Check sheet for the modelled part. Datum: model origin and axes. Units: mm. A direction names the side the tool comes from. Round coordinates to 2 decimals unless told otherwise and drop trailing zeros. Loops run counter-clockwise (first coordinate to the right, second up) from the corner with the lowest first, then second, coordinate; pieces in that order, holes last. Notation, with made-up numbers: (-6.5, 74) -> (31.5, 74) arc R22 cw to (31.5, 87) -> close; hole circle Ø5 at (15.5, 65). An arc over 180 degrees is marked (long way). One line per question, with ' | ' between items.
```python
from build123d import *

# Parameters (mm, degrees)
F1_DEPTH  = 104.648
F2_W      = 6.35
F2_H      = 4.826
F3_DEPTH  = 28.575
F5_DEPTH  = 68.58
F7_DEPTH  = 12.7
F11_DEPTH = 39.116
F12_W     = 31.242
F12_H     = 31.75
F13_DEPTH = 67.31


with BuildPart() as f1:
    # F0 (on Right) → F1 (new body)
    with BuildSketch(Plane.YZ):
        Polygon((-14.224, 15.875), (-14.224, 0), (-14.224, -15.875), (-7.874, -15.875), (-7.874, -44.45), (7.874, -44.45), (7.874, -15.875), (14.224, -15.875), (14.224, 0), (14.224, 15.875), (7.874, 15.875), (7.874, 44.45), (-7.874, 44.45), (-7.874, 15.875), align=None)
    extrude(amount=-F1_DEPTH)

    # F2 (on face) → F3 (cut, through all)
    with BuildSketch(Plane.XY.offset(44.45)):
        with Locations((-101.473, -5.461)):
            Rectangle(F2_W, F2_H)
    extrude(amount=-F3_DEPTH, mode=Mode.SUBTRACT)

    # F4 (on Front) → F5 (cut, symmetric)
    with BuildSketch(Plane.XZ):
        with BuildLine():
            Line((-50.546, -24.638), (-74.422, -24.638))
            ThreePointArc((-74.422, -24.638), (-80.01, -30.226), (-74.422, -35.814))
            Line((-74.422, -35.814), (-50.546, -35.814))
            ThreePointArc((-50.546, -35.814), (-44.958, -30.226), (-50.546, -24.638))
        make_face()
        with BuildLine():
            ThreePointArc((-74.422, 35.814), (-80.01, 30.226), (-74.422, 24.638))
            Line((-74.422, 24.638), (-50.546, 24.638))
            ThreePointArc((-50.546, 24.638), (-44.958, 30.226), (-50.546, 35.814))
            Line((-50.546, 35.814), (-74.422, 35.814))
        make_face()
    extrude(amount=F5_DEPTH, both=True, mode=Mode.SUBTRACT)


with BuildPart() as f7:
    # F6 (on Front) → F7 (new body, symmetric)
    with BuildSketch(Plane.XZ):
        Polygon((0, 44.45), (-35.052, 44.45), (-35.052, 26.924), (-17.526, 26.924), align=None)
        Polygon((0, -44.45), (-17.526, -26.924), (-35.052, -26.924), (-35.052, -44.45), align=None)
    extrude(amount=F7_DEPTH, both=True)

    # F8: union F1
    add(f1.part)

    # F10 (on Front) → F11 (cut, symmetric)
    with BuildSketch(Plane.XZ):
        Polygon((0, 44.45), (-17.526, 26.924), (-28.575, 15.875), (0, 15.875), align=None)
        Polygon((-28.575, -15.875), (-17.526, -26.924), (0, -44.45), (0, -15.875), align=None)
    extrude(amount=F11_DEPTH, both=True, mode=Mode.SUBTRACT)

    # F12 (on Front) → F13 (cut, symmetric)
    with BuildSketch(Plane.XZ):
        with Locations((-15.621, 0)):
            Rectangle(F12_W, F12_H)
    extrude(amount=F13_DEPTH, both=True, mode=Mode.SUBTRACT)


solid = f7.part
```
(1) Sectioned sample at D-D, the plane x = -12.5. Record the cut outline in (y, z).
Answer:
outline: (-12.7, -44.45) -> (12.7, -44.45) -> (12.7, -31.95) -> (-12.7, -31.95) -> close; (-12.7, 31.95) -> (12.7, 31.95) -> (12.7, 44.45) -> (-12.7, 44.45) -> close
(2) Mould release check, pull along X, two halves, no side actions. Record for faces 1 (the face through (-10.91, 0.18, 33.54)), 2 (the face through (-67, 14.224, 0)), 3 (the face through (-62, 0, -24.638)): +X half, -X half, draft (parallel to the pull), parting line (faces both ways), or undercut.
Answer:
face 1: +X half | face 2: draft | face 3: undercut
(3) Scan lines: probe 1 along Z at (x, y) = (-54.5, 4.75); probe 2 along Z at (x, y) = (-49, 0.75); probe 3 along Y at (x, z) = (-39.5, -17.5). Record each from-to range of solid material in increasing order.
Answer:
probe 1: z = -44.45 to -35.81, -24.64 to 24.64, 35.81 to 44.45 | probe 2: z = -44.45 to -35.6, -24.86 to 24.86, 35.6 to 44.45 | probe 3: y = -7.87 to 7.87
(4) Sectioned sample at B-B, the plane y = 1.75. Record the cut outline in (x, z) (3 decimals).
Answer:
outline: (-104.648, -44.45) -> (0, -44.45) -> (-28.575, -15.875) -> (-31.242, -15.875) -> (-31.242, 15.875) -> (-28.575, 15.875) -> (0, 44.45) -> (-104.648, 44.45) -> close; hole (-74.422, -35.814) -> (-50.546, -35.814) arc R5.588 ccw to (-50.546, -24.638) -> (-74.422, -24.638) arc R5.588 ccw to start; hole (-74.422, 24.638) -> (-50.546, 24.638) arc R5.588 ccw to (-50.546, 35.814) -> (-74.422, 35.814) arc R5.588 ccw to start
(5) Go/stop test with flat-tipped pins: pin 1 (1.4 mm diameter, centred on y = -9.5, z = -37.5, fed in from -X); pin 2 (10 mm diameter, centred on x = -46, z = 33.5, fed in from +Y); pin 3 (5 mm diameter, centred on x = -77, y = 11, fed in from -Z) (3 decimals); pin 4 (23 mm diameter, centred on x = -60, z = -26, fed in from -Y). Record where each tip stops, or that it passes through.
Answer:
pin 1: stops at x = -35.05 | pin 2: stops at y = 7.87 | pin 3: stops at z = -15.875 | pin 4: stops at y = -14.22
(6) Sectioned sample at C-C, the plane z = -30.5. Record the cut outline in (x, y), and give its area (3 significant figures).
Answer:
outline: (-104.65, -7.87) -> (-80, -7.87) -> (-80, 7.87) -> (-104.65, 7.87) -> close; (-44.96, -7.87) -> (-35.05, -7.87) -> (-35.05, -12.7) -> (-13.95, -12.7) -> (-13.95, 12.7) -> (-35.05, 12.7) -> (-35.05, 7.87) -> (-44.96, 7.87) -> close | area: 1,080 mm2
(7) Sectioned sample at A-A, the plane x = -68. Record the cut outline in (y, z) (3 decimals).
Answer:
outline: (-14.224, -15.875) -> (-7.874, -15.875) -> (-7.874, -24.638) -> (7.874, -24.638) -> (7.874, -15.875) -> (14.224, -15.875) -> (14.224, 15.875) -> (7.874, 15.875) -> (7.874, 24.638) -> (-7.874, 24.638) -> (-7.874, 15.875) -> (-14.224, 15.875) -> close; (-7.874, -44.45) -> (7.874, -44.45) -> (7.874, -35.814) -> (-7.874, -35.814) -> close; (-7.874, 35.814) -> (7.874, 35.814) -> (7.874, 44.45) -> (-7.874, 44.45) -> close
(8) Set-up check for faces 4 (the face through (-30, 0, -15.875)), 5 (the face through (-22, -12.7, 36)), 6 (the face through (-80.01, 0.11, -30.1)): record each of +Z, -Z, +X, -X, +Y, -Y from which the full face is reachable in a straight line by a thin tool's end or side.
Answer:
face 4: +X, +Y, -Y | face 5: +Z, +X, -X, -Y | face 6: +Y, -Y
